```python
from build123d import *

# Parameters (mm, degrees)
SKETCH_1_R          = 9.53
EXTRUDE_1_DEPTH     = 4
SKETCH_4_W          = 46.2
SKETCH_4_H          = 8.602857229
EXTRUDE_2_DEPTH     = 4
SKETCH_2_R          = 2
SKETCH_2_R_2        = 1.5
SKETCH_2_W          = 8.2
SKETCH_2_H          = 4.2
CUT_EXTRUDE_1_DEPTH = 4
CUT_EXTRUDE_2_DEPTH = 10


with BuildPart() as part:
    # 草图1 → 凸台-拉伸1 (new body)
    with BuildSketch(Plane.XY):
        with BuildLine():
            Line((328.542857143, -40.145714286), (-1.457142857, -40.145714286))
            ThreePointArc((-1.457142857, -40.145714286), (-41.457142857, -0.145714286), (-1.457142857, 39.854285714))
            Line((-1.457142857, 39.854285714), (328.542857143, 39.854285714))
            ThreePointArc((328.542857143, 39.854285714), (368.542857143, -0.145714286), (328.542857143, -40.145714286))
        make_face()
        with Locations((-1.457142857, -0.145714286)):
            Circle(SKETCH_1_R, mode=Mode.SUBTRACT)
        with Locations((328.542857143, -0.145714286)):
            Circle(SKETCH_1_R, mode=Mode.SUBTRACT)
    extrude(amount=EXTRUDE_1_DEPTH)

    # 草图4 → 凸台-拉伸2 (add)
    with BuildSketch(Plane.XY.offset(4)):
        with Locations((18.542857143, 39.652857099)):
            Rectangle(SKETCH_4_W, SKETCH_4_H)
    extrude(amount=-EXTRUDE_2_DEPTH)

    # 草图2 → 切除-拉伸1 (cut)
    with BuildSketch(Plane.XY.offset(4)):
        with Locations((108.542857143, 33.854285714)):
            Circle(SKETCH_2_R)
        with Locations((198.542857143, 33.854285714)):
            Circle(SKETCH_2_R)
        with Locations((288.542857143, 33.854285714)):
            Circle(SKETCH_2_R)
        with Locations((108.542857143, -34.145714286)):
            Circle(SKETCH_2_R)
        with Locations((198.542857143, -34.145714286)):
            Circle(SKETCH_2_R)
        with Locations((288.542857143, -34.145714286)):
            Circle(SKETCH_2_R)
        with Locations((18.542857143, -34.145714286)):
            Circle(SKETCH_2_R)
        with Locations((18.542857143, 40.014285714)):
            Circle(SKETCH_2_R_2)
        Polygon((31.542857143, -21.145714286), (104.183898028, -21.145714286), (159.772133322, 20.854285714), (31.542857143, 20.854285714), align=None)
        Polygon((275.542857143, 20.854285714), (202.901816258, 20.854285714), (147.313580964, -21.145714286), (275.542857143, -21.145714286), align=None)
        with Locations((33.542857143, 40.014285714)):
            Rectangle(SKETCH_2_W, SKETCH_2_H)
        with Locations((3.542857143, 40.014285714)):
            Rectangle(SKETCH_2_W, SKETCH_2_H)
    extrude(amount=-CUT_EXTRUDE_1_DEPTH, mode=Mode.SUBTRACT)

    # 草图3 → 切除-拉伸2 (cut)
    with BuildSketch(Plane.XY.offset(4)):
        with BuildLine():
            Line((183.145474057, 18.460683743), (155.35135641, -2.539316257))
            ThreePointArc((155.35135641, -2.539316257), (151.149255171, -1.954213553), (151.734357875, 2.247887686))
            Line((151.734357875, 2.247887686), (179.528475522, 23.247887686))
            ThreePointArc((179.528475522, 23.247887686), (183.730576762, 22.662784982), (183.145474057, 18.460683743))
        make_face()
    extrude(amount=-CUT_EXTRUDE_2_DEPTH, mode=Mode.SUBTRACT)


solid = part.part
```
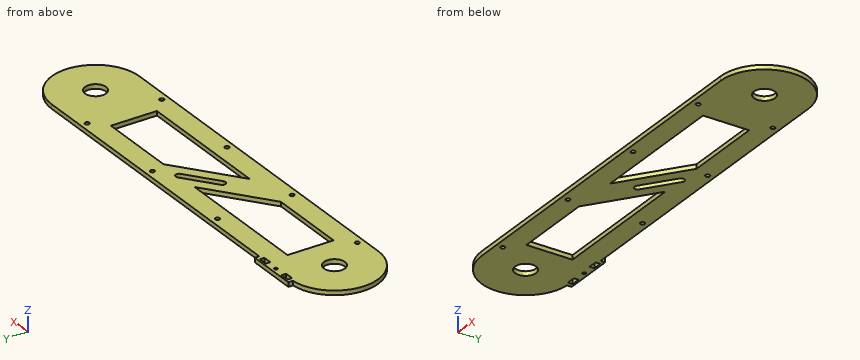
Read the model definition and answer for the solid it produces. Units are mm, in the model's axes. Round coordinates to 2 decimals unless told otherwise and drop trailing zeros. Write each loop counter-clockwise with the first axis right and the second up, starting at its lowest first coordinate (ties: lowest second). Pieces come first, ordered by that corner, then holes. Notation, with made-up numbers: (-25, -5.75) -> (-10, -5.75) arc R13 ccw to (-10, 5.25) -> close; hole circle Ø1 at (-22.5, 42.25). An arc over 180 degrees is marked (long way). Answer in a Markdown table with one row per item. Add a question column.
1) Find section C-C, the plane z = 0.8. State how many separate pieces and enclosed holes the cut face has, and give its area (3 significant figures).
2) Find section D-D, the plane x = 137.5. Determine the outline of the cut face in (y, z).
3) Find section B-B, the plane x = 4. Determine the outline of the cut face in (y, z), and give its area (3 significant figures).
4) Find section A-A, the plane x = 59.5. Determine the outline of the cut face in (y, z).
5) Given P1, Ø2, axis at y = 1.5, z = 1.5, coming from the -X side; P2, Ø2.5, axis at x = 108.54, y = -34.15, coming from the +Z side; P3, Ø1.2, axis at x = 116, z = 2.5, coming from the +Y side; P4, Ø2, axis at y = 4, z = 1.5, coming from the +X side, each flat-ended and moving along its own axis, determine where each tip first touches the part or whether it passes through.
6) Consider line 1 (Y direction, x = 257, z = 2.15); line 2 (Y direction, x = 3, z = 1.95); line 3 (X direction, y = 3, z = 1.5). Determine where each line is inside the solid, lowest interval first.
Findings below:
| question | item | result |
|---|---|---|
| 1 | separate pieces | 1 |
| 1 | enclosed holes | 15 |
| 1 | area | 22,200 mm² |
| 2 | outline | (-40.15, 0) -> (4.03, 0) -> (4.03, 4) -> (-40.15, 4) -> close; (20.85, 0) -> (39.85, 0) -> (39.85, 4) -> (20.85, 4) -> close |
| 3 | outline | (-40.15, 0) -> (-7.96, 0) -> (-7.96, 4) -> (-40.15, 4) -> close; (7.67, 0) -> (37.91, 0) -> (37.91, 4) -> (7.67, 4) -> close; (42.11, 0) -> (43.95, 0) -> (43.95, 4) -> (42.11, 4) -> close |
| 3 | area | 257 mm² |
| 4 | outline | (-40.15, 0) -> (-21.15, 0) -> (-21.15, 4) -> (-40.15, 4) -> close; (20.85, 0) -> (39.85, 0) -> (39.85, 4) -> (20.85, 4) -> close |
| 5 | P1 | x = -41.45 |
| 5 | P2 | through |
| 5 | P3 | y = 39.85 |
| 5 | P4 | x = 368.42 |
| 6 | line 1 | -40.15 to -21.15, 20.85 to 39.85 |
| 6 | line 2 | -40.15 to -8.57, 8.28 to 37.91, 42.11 to 43.95 |
| 6 | line 3 | -41.33 to -10.45, 7.54 to 31.54, 136.14 to 152.73, 162.68 to 179.27, 275.54 to 319.55, 337.54 to 368.42 |
